Source: CAD feature listing. Evaluate the final solid. Frame: model axes, mm. A direction names the side the tool comes from. Coordinates: 2 decimals unless noted, no trailing zeros. Loops run counter-clockwise (first coordinate to the right, second up) from the corner with the lowest first, then second, coordinate; pieces in that order, holes last. Notation, with made-up numbers: M 82.5,33.5 L 132.5,33.5 A31 cw 132.5,66.5 Z; hole C 15.5,64 d6. An arc over 180 degrees is marked long. One line per question, with ' | ' between items. Start each with the question number.
1. Section query C-C, the plane x = 103.5. Output: boundary loops of the cut face in (y, z), and give its area (3 significant figures).
2. Ray query, probe 1 along X at (y, z) = (9, 4.7); probe 2 along Y at (x, z) = (-11.5, 1.25); probe 3 along X at (y, z) = (-61, 4.55). Return the intervals inside material, ascending.
3. Pin query (flat end, axial travel): P1, Ø2, axis at y = -81.5, z = 3.5, coming from the -X side; P2, Ø2.5, axis at x = 145.5, z = 1.5, coming from the +Y side; P3, Ø1.5, axis at y = -69, z = 1.5, coming from the -X side. Return the tip coordinate at first contact, or that it passes through.
4. Section query A-A, the plane y = -9.5. Output: boundary loops of the cut face in (x, z), and give its area (3 significant figures).
5. Mould query, pull axis Y, two halves, no side actions, for faces 1 (the flat face through (70, -84.113, 2)), 2 (the flat face through (-39.462, -32, 3)), 3 (the flat face through (-42, 0.09, 3)), 4 (the flat face through (192.624, 13, 3)). Classes: pulls with the +Y half, pulls with the -Y half, needs draft (parallel to the pull), parting line crosses it, or undercut.
6. Section query B-B, the plane y = -67. Output: boundary loops of the cut face in (x, z), and give its area (3 significant figures).
7. Access query for faces 5 (the flat face through (222.624, 13, 3)), 6 (the flat face through (-42, -34.91, 3)), 7 (the flat face through (48, -79.717, 2)). Directions: +Z, -Z, +X, -X, +Y, -Y. A direction counts if a zero-diameter tool reaches every point of the face in a straight line with its end or side. Return the directions, or none.
```python
from build123d import *

# Parameters (mm, degrees)
ESQUISSE1_W                = 296.913296363
ESQUISSE1_H                = 99.202689883
BOSS_EXTRU_1_DEPTH         = 5
ENL_V_MAT_EXTRU_1_DEPTH    = 10
ESQUISSE3_W                = 5.229303798
ESQUISSE3_H                = 4.396229451
ENL_V_MAT_EXTRU_2_DEPTH    = 10
R_P_TITION_LIN_AIRE1_COUNT = 7
R_P_TITION_LIN_AIRE1_PITCH = 15
SYM_TRIE1_COPY_1_SKETCH_W  = 5.229303798
SYM_TRIE1_COPY_1_SKETCH_H  = 4.396229451
SYM_TRIE1_COPY_1_DEPTH     = 10
SYM_TRIE1_COPY_2_SKETCH_W  = 5.229303798
SYM_TRIE1_COPY_2_SKETCH_H  = 4.396229451
SYM_TRIE1_COPY_2_DEPTH     = 10
SYM_TRIE1_COPY_3_SKETCH_W  = 5.229303798
SYM_TRIE1_COPY_3_SKETCH_H  = 4.396229451
SYM_TRIE1_COPY_3_DEPTH     = 10
SYM_TRIE1_COPY_4_SKETCH_W  = 5.229303798
SYM_TRIE1_COPY_4_SKETCH_H  = 4.396229451
SYM_TRIE1_COPY_4_DEPTH     = 10
SYM_TRIE1_COPY_5_SKETCH_W  = 5.229303798
SYM_TRIE1_COPY_5_SKETCH_H  = 4.396229451
SYM_TRIE1_COPY_5_DEPTH     = 10
SYM_TRIE1_COPY_6_SKETCH_W  = 5.229303798
SYM_TRIE1_COPY_6_SKETCH_H  = 4.396229451
SYM_TRIE1_COPY_6_DEPTH     = 10
ESQUISSE4_W                = 58.738288448
ESQUISSE4_H                = 4.540442772
ENL_V_MAT_EXTRU_3_DEPTH    = 10
ENL_V_MAT_EXTRU_4_DEPTH    = 10
ESQUISSE6_W                = 5
ESQUISSE6_H                = 5
ENL_V_MAT_EXTRU_5_DEPTH    = 5
R_P_TITION_LIN_AIRE2_COUNT = 8
R_P_TITION_LIN_AIRE2_PITCH = 15
ESQUISSE7_W                = 57
ESQUISSE7_H                = 5
ENL_V_MAT_EXTRU_6_DEPTH    = 5
ENL_V_MAT_EXTRU_7_DEPTH    = 5
SYM_TRIE2_COPY_1_SKETCH_W  = 5
SYM_TRIE2_COPY_1_SKETCH_H  = 5
SYM_TRIE2_COPY_1_DEPTH     = 5
SYM_TRIE2_COPY_2_SKETCH_W  = 5
SYM_TRIE2_COPY_2_SKETCH_H  = 5
SYM_TRIE2_COPY_2_DEPTH     = 5
SYM_TRIE2_COPY_3_SKETCH_W  = 5
SYM_TRIE2_COPY_3_SKETCH_H  = 5
SYM_TRIE2_COPY_3_DEPTH     = 5
SYM_TRIE2_COPY_4_SKETCH_W  = 5
SYM_TRIE2_COPY_4_SKETCH_H  = 5
SYM_TRIE2_COPY_4_DEPTH     = 5
SYM_TRIE2_COPY_5_SKETCH_W  = 5
SYM_TRIE2_COPY_5_SKETCH_H  = 5
SYM_TRIE2_COPY_5_DEPTH     = 5
SYM_TRIE2_COPY_6_SKETCH_W  = 5
SYM_TRIE2_COPY_6_SKETCH_H  = 5
SYM_TRIE2_COPY_6_DEPTH     = 5
SYM_TRIE2_COPY_7_SKETCH_W  = 5
SYM_TRIE2_COPY_7_SKETCH_H  = 5
SYM_TRIE2_COPY_7_DEPTH     = 5
ESQUISSE9_W                = 4.913296363
ESQUISSE9_H                = 18.600386247
ENL_V_MAT_EXTRU_8_DEPTH    = 5
ESQUISSE10_W               = 5
ESQUISSE10_H               = 5
ENL_V_MAT_EXTRU_9_DEPTH    = 5
R_P_TITION_LIN_AIRE3_COUNT = 4
R_P_TITION_LIN_AIRE3_PITCH = 15
SYM_TRIE3_COPY_1_SKETCH_W  = 5
SYM_TRIE3_COPY_1_SKETCH_H  = 5
SYM_TRIE3_COPY_1_DEPTH     = 5
SYM_TRIE3_COPY_2_SKETCH_W  = 5
SYM_TRIE3_COPY_2_SKETCH_H  = 5
SYM_TRIE3_COPY_2_DEPTH     = 5
SYM_TRIE3_COPY_3_SKETCH_W  = 5
SYM_TRIE3_COPY_3_SKETCH_H  = 5
SYM_TRIE3_COPY_3_DEPTH     = 5


with BuildPart() as part:
    # Esquisse1 → Boss.-Extru.1 (new body)
    with BuildSketch(Plane.XY):
        with Locations((104.081072913, -34.511559996)):
            Rectangle(ESQUISSE1_W, ESQUISSE1_H)
    extrude(amount=BOSS_EXTRU_1_DEPTH)

    # Esquisse2 → Enlèv. mat.-Extru.1 (cut)
    with BuildSketch(Plane(origin=(0, 0, 0), x_dir=(-1, 0, 0), z_dir=(0, 0, -1))):
        Polygon((44.375575269, -78.510601301), (39.375575269, -78.510601301), (37.504666451, -84.112904937), (44.375575269, -84.112904937), align=None)
    enl_v_mat_extru_1 = extrude(amount=-ENL_V_MAT_EXTRU_1_DEPTH, mode=Mode.SUBTRACT)

    # Esquisse3 → Enlèv. mat.-Extru.2 (cut)
    with BuildSketch(Plane(origin=(0, 0, 0), x_dir=(-1, 0, 0), z_dir=(0, 0, -1))):
        with Locations((26.890031572, -81.914790212)):
            Rectangle(ESQUISSE3_W, ESQUISSE3_H)
    enl_v_mat_extru_2 = extrude(amount=-ENL_V_MAT_EXTRU_2_DEPTH, mode=Mode.SUBTRACT)

    # Répétition linéaire1: Enlèv. mat.-Extru.2 ×7
    with Locations(*[(i * R_P_TITION_LIN_AIRE1_PITCH, 0, 0) for i in range(1, R_P_TITION_LIN_AIRE1_COUNT)]):
        add(enl_v_mat_extru_2, mode=Mode.SUBTRACT)

    # Symétrie1: Enlèv. mat.-Extru.1, Enlèv. mat.-Extru.2 across plane
    add(enl_v_mat_extru_1.mirror(Plane.ZY.offset(-104.081072913)), mode=Mode.SUBTRACT)
    add(enl_v_mat_extru_2.mirror(Plane.ZY.offset(-104.081072913)), mode=Mode.SUBTRACT)

    # Symétrie1 copy 1 sketch → Symétrie1 copy 1 (cut)
    with BuildSketch(Plane(origin=(193.162145825, 0, 0), x_dir=(1, 0, 0), z_dir=(0, 0, -1))):
        with Locations((26.890031572, 81.914790212)):
            Rectangle(SYM_TRIE1_COPY_1_SKETCH_W, SYM_TRIE1_COPY_1_SKETCH_H)
    extrude(amount=-SYM_TRIE1_COPY_1_DEPTH, mode=Mode.SUBTRACT)

    # Symétrie1 copy 2 sketch → Symétrie1 copy 2 (cut)
    with BuildSketch(Plane(origin=(178.162145825, 0, 0), x_dir=(1, 0, 0), z_dir=(0, 0, -1))):
        with Locations((26.890031572, 81.914790212)):
            Rectangle(SYM_TRIE1_COPY_2_SKETCH_W, SYM_TRIE1_COPY_2_SKETCH_H)
    extrude(amount=-SYM_TRIE1_COPY_2_DEPTH, mode=Mode.SUBTRACT)

    # Symétrie1 copy 3 sketch → Symétrie1 copy 3 (cut)
    with BuildSketch(Plane(origin=(163.162145825, 0, 0), x_dir=(1, 0, 0), z_dir=(0, 0, -1))):
        with Locations((26.890031572, 81.914790212)):
            Rectangle(SYM_TRIE1_COPY_3_SKETCH_W, SYM_TRIE1_COPY_3_SKETCH_H)
    extrude(amount=-SYM_TRIE1_COPY_3_DEPTH, mode=Mode.SUBTRACT)

    # Symétrie1 copy 4 sketch → Symétrie1 copy 4 (cut)
    with BuildSketch(Plane(origin=(148.162145825, 0, 0), x_dir=(1, 0, 0), z_dir=(0, 0, -1))):
        with Locations((26.890031572, 81.914790212)):
            Rectangle(SYM_TRIE1_COPY_4_SKETCH_W, SYM_TRIE1_COPY_4_SKETCH_H)
    extrude(amount=-SYM_TRIE1_COPY_4_DEPTH, mode=Mode.SUBTRACT)

    # Symétrie1 copy 5 sketch → Symétrie1 copy 5 (cut)
    with BuildSketch(Plane(origin=(133.162145825, 0, 0), x_dir=(1, 0, 0), z_dir=(0, 0, -1))):
        with Locations((26.890031572, 81.914790212)):
            Rectangle(SYM_TRIE1_COPY_5_SKETCH_W, SYM_TRIE1_COPY_5_SKETCH_H)
    extrude(amount=-SYM_TRIE1_COPY_5_DEPTH, mode=Mode.SUBTRACT)

    # Symétrie1 copy 6 sketch → Symétrie1 copy 6 (cut)
    with BuildSketch(Plane(origin=(118.162145825, 0, 0), x_dir=(1, 0, 0), z_dir=(0, 0, -1))):
        with Locations((26.890031572, 81.914790212)):
            Rectangle(SYM_TRIE1_COPY_6_SKETCH_W, SYM_TRIE1_COPY_6_SKETCH_H)
    extrude(amount=-SYM_TRIE1_COPY_6_DEPTH, mode=Mode.SUBTRACT)

    # Esquisse4 → Enlèv. mat.-Extru.3 (cut)
    with BuildSketch(Plane(origin=(0, 0, 0), x_dir=(-1, 0, 0), z_dir=(0, 0, -1))):
        with Locations((-104.051236875, -81.842683551)):
            Rectangle(ESQUISSE4_W, ESQUISSE4_H)
    extrude(amount=-ENL_V_MAT_EXTRU_3_DEPTH, mode=Mode.SUBTRACT)

    # Esquisse5 → Enlèv. mat.-Extru.4 (cut)
    with BuildSketch(Plane(origin=(0, 0, 0), x_dir=(-1, 0, 0), z_dir=(0, 0, -1))):
        with BuildLine():
            Line((-74.682092651, -79.572462165), (-133.420381099, -79.572462165))
            ThreePointArc((-133.420381099, -79.572462165), (-104.051236875, -50.20331794), (-74.682092651, -79.572462165))
        make_face()
    extrude(amount=-ENL_V_MAT_EXTRU_4_DEPTH, mode=Mode.SUBTRACT)

    # Esquisse6 → Enlèv. mat.-Extru.5 (cut)
    with BuildSketch(Plane.XY.offset(5)):
        with Locations((235.124424731, 12.589784946)):
            Rectangle(ESQUISSE6_W, ESQUISSE6_H)
    enl_v_mat_extru_5 = extrude(amount=-ENL_V_MAT_EXTRU_5_DEPTH, mode=Mode.SUBTRACT)

    # Répétition linéaire2: Enlèv. mat.-Extru.5 ×8
    with Locations(*[(-i * R_P_TITION_LIN_AIRE2_PITCH, 0, 0) for i in range(1, R_P_TITION_LIN_AIRE2_COUNT)]):
        add(enl_v_mat_extru_5, mode=Mode.SUBTRACT)

    # Esquisse7 → Enlèv. mat.-Extru.6 (cut)
    with BuildSketch(Plane.XY.offset(5)):
        with Locations((104.124424731, 12.589784946)):
            Rectangle(ESQUISSE7_W, ESQUISSE7_H)
    extrude(amount=-ENL_V_MAT_EXTRU_6_DEPTH, mode=Mode.SUBTRACT)

    # Esquisse8 → Enlèv. mat.-Extru.7 (cut)
    with BuildSketch(Plane.XY.offset(5)):
        with BuildLine():
            ThreePointArc((132.624424731, 10.089784946), (104.124424731, -18.410215054), (75.624424731, 10.089784946))
            Line((75.624424731, 10.089784946), (132.624424731, 10.089784946))
        make_face()
    extrude(amount=-ENL_V_MAT_EXTRU_7_DEPTH, mode=Mode.SUBTRACT)

    # Symétrie2: Enlèv. mat.-Extru.5 across plane
    add(enl_v_mat_extru_5.mirror(Plane(origin=(104.081072913, 0, 0), x_dir=(0, 0, 1), z_dir=(1, 0, 0))), mode=Mode.SUBTRACT)

    # Symétrie2 copy 1 sketch → Symétrie2 copy 1 (cut)
    with BuildSketch(Plane(origin=(223.162145825, 0, 5), x_dir=(-1, 0, 0), z_dir=(0, 0, 1))):
        with Locations((235.124424731, -12.589784946)):
            Rectangle(SYM_TRIE2_COPY_1_SKETCH_W, SYM_TRIE2_COPY_1_SKETCH_H)
    extrude(amount=-SYM_TRIE2_COPY_1_DEPTH, mode=Mode.SUBTRACT)

    # Symétrie2 copy 2 sketch → Symétrie2 copy 2 (cut)
    with BuildSketch(Plane(origin=(238.162145825, 0, 5), x_dir=(-1, 0, 0), z_dir=(0, 0, 1))):
        with Locations((235.124424731, -12.589784946)):
            Rectangle(SYM_TRIE2_COPY_2_SKETCH_W, SYM_TRIE2_COPY_2_SKETCH_H)
    extrude(amount=-SYM_TRIE2_COPY_2_DEPTH, mode=Mode.SUBTRACT)

    # Symétrie2 copy 3 sketch → Symétrie2 copy 3 (cut)
    with BuildSketch(Plane(origin=(253.162145825, 0, 5), x_dir=(-1, 0, 0), z_dir=(0, 0, 1))):
        with Locations((235.124424731, -12.589784946)):
            Rectangle(SYM_TRIE2_COPY_3_SKETCH_W, SYM_TRIE2_COPY_3_SKETCH_H)
    extrude(amount=-SYM_TRIE2_COPY_3_DEPTH, mode=Mode.SUBTRACT)

    # Symétrie2 copy 4 sketch → Symétrie2 copy 4 (cut)
    with BuildSketch(Plane(origin=(268.162145825, 0, 5), x_dir=(-1, 0, 0), z_dir=(0, 0, 1))):
        with Locations((235.124424731, -12.589784946)):
            Rectangle(SYM_TRIE2_COPY_4_SKETCH_W, SYM_TRIE2_COPY_4_SKETCH_H)
    extrude(amount=-SYM_TRIE2_COPY_4_DEPTH, mode=Mode.SUBTRACT)

    # Symétrie2 copy 5 sketch → Symétrie2 copy 5 (cut)
    with BuildSketch(Plane(origin=(283.162145825, 0, 5), x_dir=(-1, 0, 0), z_dir=(0, 0, 1))):
        with Locations((235.124424731, -12.589784946)):
            Rectangle(SYM_TRIE2_COPY_5_SKETCH_W, SYM_TRIE2_COPY_5_SKETCH_H)
    extrude(amount=-SYM_TRIE2_COPY_5_DEPTH, mode=Mode.SUBTRACT)

    # Symétrie2 copy 6 sketch → Symétrie2 copy 6 (cut)
    with BuildSketch(Plane(origin=(298.162145825, 0, 5), x_dir=(-1, 0, 0), z_dir=(0, 0, 1))):
        with Locations((235.124424731, -12.589784946)):
            Rectangle(SYM_TRIE2_COPY_6_SKETCH_W, SYM_TRIE2_COPY_6_SKETCH_H)
    extrude(amount=-SYM_TRIE2_COPY_6_DEPTH, mode=Mode.SUBTRACT)

    # Symétrie2 copy 7 sketch → Symétrie2 copy 7 (cut)
    with BuildSketch(Plane(origin=(313.162145825, 0, 5), x_dir=(-1, 0, 0), z_dir=(0, 0, 1))):
        with Locations((235.124424731, -12.589784946)):
            Rectangle(SYM_TRIE2_COPY_7_SKETCH_W, SYM_TRIE2_COPY_7_SKETCH_H)
    extrude(amount=-SYM_TRIE2_COPY_7_DEPTH, mode=Mode.SUBTRACT)

    # Esquisse9 → Enlèv. mat.-Extru.8 (cut)
    with BuildSketch(Plane.XY.offset(5)):
        with Locations((250.081072913, -69.210408177)):
            Rectangle(ESQUISSE9_W, ESQUISSE9_H)
    enl_v_mat_extru_8 = extrude(amount=-ENL_V_MAT_EXTRU_8_DEPTH, mode=Mode.SUBTRACT)

    # Esquisse10 → Enlèv. mat.-Extru.9 (cut)
    with BuildSketch(Plane.XY.offset(5)):
        with Locations((250.124424731, -47.410215054)):
            Rectangle(ESQUISSE10_W, ESQUISSE10_H)
    enl_v_mat_extru_9 = extrude(amount=-ENL_V_MAT_EXTRU_9_DEPTH, mode=Mode.SUBTRACT)

    # Répétition linéaire3: Enlèv. mat.-Extru.9 ×4
    with Locations(*[(0, i * R_P_TITION_LIN_AIRE3_PITCH, 0) for i in range(1, R_P_TITION_LIN_AIRE3_COUNT)]):
        add(enl_v_mat_extru_9, mode=Mode.SUBTRACT)

    # Symétrie3: Enlèv. mat.-Extru.8, Enlèv. mat.-Extru.9 across plane
    add(enl_v_mat_extru_8.mirror(Plane(origin=(104.081072913, 0, 0), x_dir=(0, 0, 1), z_dir=(1, 0, 0))), mode=Mode.SUBTRACT)
    add(enl_v_mat_extru_9.mirror(Plane(origin=(104.081072913, 0, 0), x_dir=(0, 0, 1), z_dir=(1, 0, 0))), mode=Mode.SUBTRACT)

    # Symétrie3 copy 1 sketch → Symétrie3 copy 1 (cut)
    with BuildSketch(Plane(origin=(208.162145825, 15, 5), x_dir=(-1, 0, 0), z_dir=(0, 0, 1))):
        with Locations((250.124424731, 47.410215054)):
            Rectangle(SYM_TRIE3_COPY_1_SKETCH_W, SYM_TRIE3_COPY_1_SKETCH_H)
    extrude(amount=-SYM_TRIE3_COPY_1_DEPTH, mode=Mode.SUBTRACT)

    # Symétrie3 copy 2 sketch → Symétrie3 copy 2 (cut)
    with BuildSketch(Plane(origin=(208.162145825, 30, 5), x_dir=(-1, 0, 0), z_dir=(0, 0, 1))):
        with Locations((250.124424731, 47.410215054)):
            Rectangle(SYM_TRIE3_COPY_2_SKETCH_W, SYM_TRIE3_COPY_2_SKETCH_H)
    extrude(amount=-SYM_TRIE3_COPY_2_DEPTH, mode=Mode.SUBTRACT)

    # Symétrie3 copy 3 sketch → Symétrie3 copy 3 (cut)
    with BuildSketch(Plane(origin=(208.162145825, 45, 5), x_dir=(-1, 0, 0), z_dir=(0, 0, 1))):
        with Locations((250.124424731, 47.410215054)):
            Rectangle(SYM_TRIE3_COPY_3_SKETCH_W, SYM_TRIE3_COPY_3_SKETCH_H)
    extrude(amount=-SYM_TRIE3_COPY_3_DEPTH, mode=Mode.SUBTRACT)


solid = part.part
```
Taken from the geometry:
1) outline: M -50.21,0 L -18.4,0 L -18.4,5 L -50.21,5 Z | area: 159 mm^2
2) probe 1: -44.38 to 75.65, 132.6 to 252.54 | probe 2: -79.72 to 10.09 | probe 3: -39.46 to 81.3, 126.8 to 247.62
3) P1: x = -38.71 | P2: y = 10.09 | P3: x = -39.46
4) outline: M -44.38,0 L 83.42,0 L 83.42,5 L -44.38,5 Z; M 124.82,0 L 252.54,0 L 252.54,5 L 124.82,5 Z | area: 1,280 mm^2
5) face 1: pulls with the -Y half | face 2: undercut | face 3: undercut | face 4: needs draft
6) outline: M -39.46,0 L 77.51,0 L 77.51,5 L -39.46,5 Z; M 130.59,0 L 247.62,0 L 247.62,5 L 130.59,5 Z | area: 1,170 mm^2
7) face 5: +Z, -Z, +Y | face 6: +Z, -Z, -X | face 7: +Z, -Z, -Y
